```python
from build123d import *

# Parameters (mm, degrees)
SKETCH1_W           = 114.3
SKETCH1_H           = 114.3
SKETCH1_R           = 3.175
BOSS_EXTRUDE2_DEPTH = 1.5875


with BuildPart() as part:
    # Sketch1 → Boss-Extrude2 (new, symmetric)
    with BuildSketch(Plane.XY):
        Rectangle(SKETCH1_W, SKETCH1_H)
        with Locations((-49.53, 44.45)):
            Circle(SKETCH1_R, mode=Mode.SUBTRACT)
        with BuildLine():
            Line((-24.425187853, -48.517802544), (24.425187853, -48.517802544))
            ThreePointArc((24.425187853, -48.517802544), (26.771841866, -46.949818462), (26.221239077, -44.181751319))
            Line((26.221239077, -44.181751319), (1.796051224, -19.756563466))
            ThreePointArc((1.796051224, -19.756563466), (0, -19.012614691), (-1.796051224, -19.756563466))
            Line((-1.796051224, -19.756563466), (-26.221239077, -44.181751319))
            ThreePointArc((-26.221239077, -44.181751319), (-26.771841866, -46.949818462), (-24.425187853, -48.517802544))
        make_face(mode=Mode.SUBTRACT)
        with BuildLine():
            Line((-48.517802544, 24.425187853), (-48.517802544, -24.425187853))
            ThreePointArc((-48.517802544, -24.425187853), (-46.949818462, -26.771841866), (-44.181751319, -26.221239077))
            Line((-44.181751319, -26.221239077), (-19.756563466, -1.796051224))
            ThreePointArc((-19.756563466, -1.796051224), (-19.012614691, 0), (-19.756563466, 1.796051224))
            Line((-19.756563466, 1.796051224), (-44.181751319, 26.221239077))
            ThreePointArc((-44.181751319, 26.221239077), (-46.949818462, 26.771841866), (-48.517802544, 24.425187853))
        make_face(mode=Mode.SUBTRACT)
        with BuildLine():
            Line((24.425187853, 48.517802544), (-24.425187853, 48.517802544))
            ThreePointArc((-24.425187853, 48.517802544), (-26.771841866, 46.949818462), (-26.221239077, 44.181751319))
            Line((-26.221239077, 44.181751319), (-1.796051224, 19.756563466))
            ThreePointArc((-1.796051224, 19.756563466), (0, 19.012614691), (1.796051224, 19.756563466))
            Line((1.796051224, 19.756563466), (26.221239077, 44.181751319))
            ThreePointArc((26.221239077, 44.181751319), (26.771841866, 46.949818462), (24.425187853, 48.517802544))
        make_face(mode=Mode.SUBTRACT)
        with BuildLine():
            Line((48.517802544, -24.425187853), (48.517802544, 24.425187853))
            ThreePointArc((48.517802544, 24.425187853), (46.949818462, 26.771841866), (44.181751319, 26.221239077))
            Line((44.181751319, 26.221239077), (19.756563466, 1.796051224))
            ThreePointArc((19.756563466, 1.796051224), (19.012614691, 0), (19.756563466, -1.796051224))
            Line((19.756563466, -1.796051224), (44.181751319, -26.221239077))
            ThreePointArc((44.181751319, -26.221239077), (46.949818462, -26.771841866), (48.517802544, -24.425187853))
        make_face(mode=Mode.SUBTRACT)
    extrude(amount=BOSS_EXTRUDE2_DEPTH, both=True)


solid = part.part
```
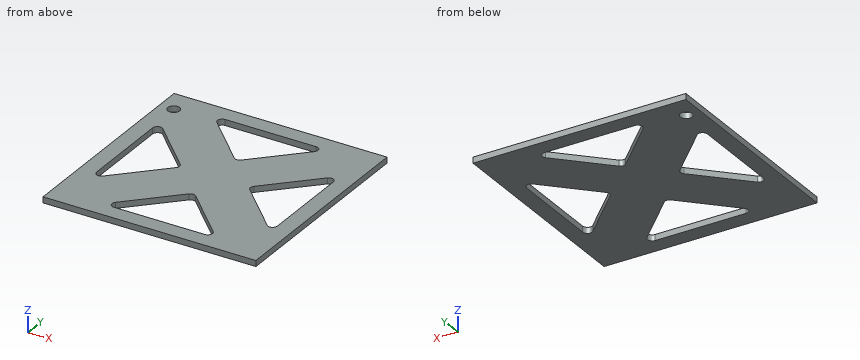
Source: CAD feature listing. Evaluate the final solid. Frame: model axes, mm. Round coordinates to 2 decimals unless told otherwise and drop trailing zeros. Write each loop counter-clockwise with the first axis right and the second up, starting at its lowest first coordinate (ties: lowest second). Pieces come first, ordered by that corner, then holes. Notation, with made-up numbers: M -19.5,-19.75 L 29.5,-19.75 A15 ccw 29.5,-15.75 Z; hole C 2,55 d7. An arc over 180 degrees is marked long. Answer as a JSON object with one key per item and string values. Group by question number.
(1) Section query D-D on x = -29. Output: boundary loops of the cut face in (y, z), then the cut area to 3 significant figures.
(2) Section query A-A on y = 10. Output: boundary loops of the cut face in (x, z), then the cut area to 3 significant figures.
(3) First-contact query: pin 1 (10 mm diameter, centred on x = -49.53, y = 44.45, fed in from +Z). Flat tip, straight axial feed; report the tip coordinate or a pass-through.
(4) Section query B-B on z = 0.1. State how many separate pieces and enclosed holes the cut face has, then the cut area to 3 significant figures.
(5) Section query C-C on x = 8.5. Output: boundary loops of the cut face in (y, z), then the cut area to 3 significant figures.
(6) Ray query, line 1 (Y direction, x = -49.53, z = 0.3) (3 decimals); line 2 (X direction, y = 0.5, z = -0.45); line 3 (Y direction, x = 1, z = 0.6). Return the intervals inside material, ascending. Write a range as [from, to].
Computed values:
{
 "1": {"outline": "M -57.15,-1.59 L -11.04,-1.59 L -11.04,1.59 L -57.15,1.59 Z; M 11.04,-1.59 L 57.15,-1.59 L 57.15,1.59 L 11.04,1.59 Z", "area": "293 mm^2"},
 "2": {"outline": "M -57.15,-1.59 L -48.52,-1.59 L -48.52,1.59 L -57.15,1.59 Z; M -27.96,-1.59 L 27.96,-1.59 L 27.96,1.59 L -27.96,1.59 Z; M 48.52,-1.59 L 57.15,-1.59 L 57.15,1.59 L 48.52,1.59 Z", "area": "232 mm^2"},
 "3": {"pin 1": "z = 1.59"},
 "4": {"separate pieces": "1", "enclosed holes": "5", "area": "9,370 mm^2"},
 "5": {"outline": "M -57.15,-1.59 L -48.52,-1.59 L -48.52,1.59 L -57.15,1.59 Z; M -26.46,-1.59 L 26.46,-1.59 L 26.46,1.59 L -26.46,1.59 Z; M 48.52,-1.59 L 57.15,-1.59 L 57.15,1.59 L 48.52,1.59 Z", "area": "223 mm^2"},
 "6": {"line 1": "[-57.15, 41.275], [47.625, 57.15]", "line 2": "[-57.15, -48.52], [-19.06, 19.06], [48.52, 57.15]", "line 3": "[-57.15, -48.52], [-19.22, 19.22], [48.52, 57.15]"}
}
